Read the model definition and answer for the solid it produces. Units are mm, in the model's axes. Face numbers are marked on the shaded views. A direction names the side the tool comes from. Give positions to 0.01 mm unless a question says otherwise; leave off trailing zeros. Order: outer loops, then holes, each group sorted by start corner. A loop starts at its lowest first (then second) coordinate and runs counter-clockwise, first axis right, second up. Notation, with made-up numbers: (27, -35) - (54, -35) arc R30 cw to (54, -2) - close; hole circle Ø7 at (-7, -33). An arc over 180 degrees is marked (long way). Use a Markdown table: item, result. Add a question column.
1. Consider L1, parallel to X at y = 0, z = 8.3; L2, parallel to Y at x = -41, z = 9 (1 decimal); L3, parallel to X at y = -1.5, z = 1.25. Determine where each line is inside the solid, lowest interval first.
2. Flat-ended cylindrical pins translate along their axes: P1, Ø4.5, axis at x = -16.59, y = 2.11, coming from the +Z side (3 decimals); P2, Ø3.5, axis at x = -41.5, y = -15.5, coming from the -Z side; P3, Ø3, axis at y = 8, z = 12, coming from the -X side. Find the tip coordinate at first contact, or state that the pin passes through.
3. A cutting plane is placed at A-A on z = 9.75. Determine the outline of the cut face in (x, y) (1 decimal).
4. Which of the six approach directions +Z, -Z, +X, -X, +Y, -Y give full straight-line access (tool end or side, diameter ignored) to the marked faces 1, 2, 3 and 4?
5. A cutting plane is placed at B-B on y = 3.5. Determine the outline of the cut face in (x, z) (1 decimal), and give its area (3 significant figures).
6. A cutting plane is placed at C-C on x = -49. Determine the outline of the cut face in (y, z) (1 decimal), and give its area (3 significant figures).
Autodesk Inventor part; units mm, degrees
ref_plane "Work Plane2" through (-20.9694, -2.2685, 9.225) normal (0, 0, -1) x (0.1078, 0.9942, 0)
ref_plane "Work Plane3" through (-49.3551, -24.0887, 15.745) normal (0, 0, -1) x (0, 1, 0)
ref_plane "Work Plane4" through (-51.466, -24.0887, 15.745) normal (0, 0, -1) x (0, 1, 0)
ref_plane "Work Plane5" through (0, 0, 0) normal (0, 0, 1) x (1, 0, 0)
sketch "Sketch1" plane through (0, 0, 0) normal (0, 0, 1) x (1, 0, 0)
  line L0 (-46.1271, -22.5825) -> (-26.1271, -22.5825) construction
  line L1 (-9.7566, 12.6962) -> (-9.7566, -12.6962) construction
  line L2 (-26.1271, 20.28) -> (-46.1271, 20.28) construction
  circle A0 centre (-49.897, 0) radius 1.778
  arc A1 (-26.7903, 1.7468) -> (-25.506, 1.3298) centre (-26.6476, 0) ccw construction
  circle A2 centre (-49.897, 0) radius 1.905
  circle A3 centre (-26.6476, 0) radius 1.905
  line L3 (-52.9366, 6.2882) -> (-52.9366, -15.9368)
  line L4 (-55.4766, 6.2882) -> (-55.4766, -15.9368) construction
  line L5 (-9.7566, -22.5825) -> (-55.4766, -22.5825)
  line L6 (-55.4766, -22.5825) -> (-55.4766, 20.28)
  line L7 (-55.4766, 20.28) -> (-9.7566, 20.28)
  line L8 (-9.7566, 20.28) -> (-9.7566, -22.5825)
  circle A4 centre (-16.5926, 2.1082) radius 2.15 construction
  circle A5 centre (-16.5926, 2.1082) radius 1.9939
  point P0 (0, 0)
  dimension "d0" = 3.81
  dimension "d1" = 3.81
  dimension "d2" = 2.54
  dimension "d3" = 3.9878
ref_plane "Work Plane2" through (-20.9694, -2.2685, 9.225) normal (0, 0, -1) x (0.1078, 0.9942, 0)
extrude "Extrusion1" add sketch "Sketch1" along normal up to surface (9.225 mm away) contours A2 | L5 L6 L7 L8
ref_plane "Work Plane3" through (-49.3551, -24.0887, 15.745) normal (0, 0, -1) x (0, 1, 0)
ref_plane "Work Plane7" through (-55.4766, -22.5825, 9.225) normal (0, 0, 1) x (1, 0, 0)
sketch "Sketch3" plane through (-55.4766, -22.5825, 9.225) normal (0, 0, 1) x (1, 0, 0)
  line L0 (27.2386, 42.8625) -> (7.2386, 42.8625)
  arc A0 (27.2386, 28.0707) -> (27.2386, 14.6543) centre (29.2386, 21.3625) ccw
  line L1 (27.2386, 0) -> (27.2386, 14.6543)
  line L2 (7.2386, 14.6543) -> (7.2386, 0)
  line L3 (7.2386, 0) -> (27.2386, 0)
  arc A1 (7.2386, 14.6543) -> (7.2386, 28.0707) centre (5.2386, 21.3625) ccw
  line L4 (7.2386, 28.0707) -> (7.2386, 42.8625)
  line L5 (0, 42.8625) -> (45.72, 42.8625)
  line L6 (27.2386, 28.0707) -> (27.2386, 42.8625)
  point P0 (55.4766, 22.5825)
ref_plane "Work Plane4" through (-51.466, -24.0887, 15.745) normal (0, 0, -1) x (0, 1, 0)
extrude "Extrusion3" add sketch "Sketch3" along normal up to surface (6.52 mm away)
ref_plane "Work Plane9" through (-55.4766, -22.5825, 9.225) normal (0, 0, 1) x (1, 0, 0)
sketch "Sketch4" plane through (-55.4766, -22.5825, 9.225) normal (0, 0, 1) x (1, 0, 0)
  circle A0 centre (5.5796, 22.5825) radius 1.778
  circle A1 centre (5.5796, 22.5825) radius 1.905
  line L0 (7.2386, 28.0707) -> (7.2386, 42.8625)
  line L1 (7.2386, 42.8625) -> (0, 42.8625)
  line L2 (0, 42.8625) -> (0, 0)
  line L3 (0, 0) -> (7.2386, 0)
  line L4 (7.2386, 0) -> (7.2386, 14.6543)
  arc A2 (7.2386, 14.6543) -> (7.2386, 28.0707) centre (5.2386, 21.3625) ccw
  circle A3 centre (5.5796, 22.5825) radius 1.778
  circle A4 centre (28.829, 22.5825) radius 1.9812
  point P0 (55.4766, 22.5825)
  dimension "d18" = 3.81
hole "Hole1" at (-49.897, 0, 9.225) at (-26.6476, 0, 9.225) direction (0, 0, -1) diameter 3.81 end through all counterbore diameter 10.16 counterbore depth 1.524
ref_plane "Work Plane8" through (-9.7566, -22.5825, 0) normal (1, 0, 0) x (0, 0, -1)
sketch "Sketch6" plane through (-9.7566, -22.5825, 0) normal (1, 0, 0) x (0, 0, -1)
  line L0 (-11.975, 30.2275) -> (-14.475, 30.2275) construction
  line L1 (-11.975, 39.7275) -> (-11.975, 30.2275) construction
  line L2 (31.025, 39.7275) -> (-11.975, 39.7275) construction
  line L3 (31.025, 38.4575) -> (-10.705, 38.4575) construction
  line L4 (-10.705, 32.1075) -> (-10.705, 28.9575) construction
  line L5 (-10.705, 28.9575) -> (-14.475, 28.9575) construction
  line L6 (-10.705, 28.9575) -> (-10.705, 32.1075)
  line L7 (0, 42.8625) -> (0, 0)
  line L8 (0, 32.1075) -> (0, 42.8625)
  line L9 (0, 42.8625) -> (-15.745, 42.8625)
  line L10 (-15.745, 42.8625) -> (-15.745, 28.9575)
  line L11 (-15.745, 28.9575) -> (-10.705, 28.9575)
  line L12 (3.1182, 32.1075) -> (5.3958, 32.1075) construction
  line L13 (-10.705, 32.1075) -> (0, 32.1075)
  point P0 (0, 22.5825)
  point P1 (0, 38.4575)
  dimension "d28" = 1.27
extrude "Extrusion4" cut sketch "Sketch6" against normal through all
sketch "Sketch7" plane through (-48.238, -22.5825, 15.745) normal (0, 0, 1) x (1, 0, 0)
  circle A0 centre (6, 5.3625) radius 2 construction
  circle A1 centre (14, 5.3625) radius 2 construction
  arc A2 (7.4142, 14.7767) -> (4.5858, 11.9483) centre (6, 13.3625) ccw construction
  arc A3 (15.4142, 11.9483) -> (12.5858, 14.7767) centre (14, 13.3625) ccw construction
  point P0 (48.238, 22.5825)
sketch "Sketch9" plane through (0, 0, 0) normal (0, 0, -1) x (-1, 0, 0)
  arc A0 (43.6522, -10.6342) -> (40.8238, -7.8058) centre (42.238, -9.22) ccw construction
  arc A1 (35.6522, -7.8058) -> (32.8238, -10.6342) centre (34.238, -9.22) ccw construction
  circle A2 centre (42.238, -17.22) radius 2 construction
  circle A3 centre (34.238, -17.22) radius 2 construction
  point P0 (0, 0)
hole "Hole2" at (-34.238, -9.22, 0) at (-42.238, -9.22, 0) at (-42.238, -17.22, 0) at (-34.238, -17.22, 0) direction (0, 0, 1) diameter 3.9878 end through all
ref_plane "Work Plane6" through (0, 0, 0) normal (0, 0, -1) x (-1, 0, 0)
sketch "Sketch10" plane through (0, 0, 0) normal (0, 0, -1) x (-1, 0, 0)
  circle A0 centre (34.238, -9.22) radius 1.9939 construction
  circle A1 centre (42.238, -9.22) radius 1.9939 construction
  circle A2 centre (42.238, -17.22) radius 1.9939 construction
  circle A3 centre (34.238, -17.22) radius 1.9939 construction
  circle A4 centre (34.238, -9.22) radius 4.2545 construction
  circle A5 centre (42.238, -9.22) radius 4.2545 construction
  line L0 (34.238, -13.4745) -> (30.5535, -11.3472)
  line L1 (30.5535, -11.3472) -> (30.5535, -7.0927)
  line L2 (30.5535, -7.0927) -> (34.238, -4.9655)
  line L3 (34.238, -4.9655) -> (37.9225, -7.0927)
  line L4 (37.9225, -7.0927) -> (37.9225, -11.3472)
  line L5 (37.9225, -11.3472) -> (34.238, -13.4745)
  circle A6 centre (34.238, -17.22) radius 4.2545 construction
  circle A7 centre (42.238, -17.22) radius 4.2545 construction
  line L6 (38.4925, -17.22) -> (36.3652, -20.9045)
  line L7 (36.3652, -20.9045) -> (32.1107, -20.9045)
  line L8 (32.1107, -20.9045) -> (29.9835, -17.22)
  line L9 (29.9835, -17.22) -> (32.1107, -13.5355)
  line L10 (32.1107, -13.5355) -> (36.3652, -13.5355)
  line L11 (36.3652, -13.5355) -> (38.4925, -17.22)
  line L12 (42.238, -21.4745) -> (38.5535, -19.3472)
  line L13 (38.5535, -19.3472) -> (38.5535, -15.0927)
  line L14 (38.5535, -15.0927) -> (42.238, -12.9655)
  line L15 (42.238, -12.9655) -> (45.9225, -15.0927)
  line L16 (45.9225, -15.0927) -> (45.9225, -19.3472)
  line L17 (45.9225, -19.3472) -> (42.238, -21.4745)
  line L18 (46.4925, -9.22) -> (44.3652, -12.9045)
  line L19 (44.3652, -12.9045) -> (40.1107, -12.9045)
  line L20 (40.1107, -12.9045) -> (37.9835, -9.22)
  line L21 (37.9835, -9.22) -> (40.1107, -5.5355)
  line L22 (40.1107, -5.5355) -> (44.3652, -5.5355)
  line L23 (44.3652, -5.5355) -> (46.4925, -9.22)
  circle A8 centre (16.5926, 2.1082) radius 1.9939 construction
  circle A9 centre (16.5926, 2.1082) radius 4.2545 construction
  line L24 (16.5926, -2.1463) -> (12.9081, -0.019)
  line L25 (12.9081, -0.019) -> (12.9081, 4.2355)
  line L26 (12.9081, 4.2355) -> (16.5926, 6.3627)
  line L27 (16.5926, 6.3627) -> (20.2771, 4.2355)
  line L28 (20.2771, 4.2355) -> (20.2771, -0.019)
  line L29 (20.2771, -0.019) -> (16.5926, -2.1463)
  point P0 (0, 0)
  point P1 (42.238, -13.4745)
  dimension "d38" = 8.509
  dimension "d44" = 8.509
  dimension "d45" = 8.509
  dimension "d48" = 8.509
  dimension "d39" = 8.509
extrude "Extrusion6" cut sketch "Sketch10" against normal blind 5.588 contours L0 L1 L2 L3 L4 L5 | L6 L7 L8 L9 L10 L11 | L12 L13 L14 L15 L16 L17 | L18 L19 L20 L21 L22 L23
extrude "Extrusion7" cut sketch "Sketch10" against normal blind 5.588 contours L24 L25 L26 L27 L28 L29
properties part number "CollectorArmRollerSupportRight"
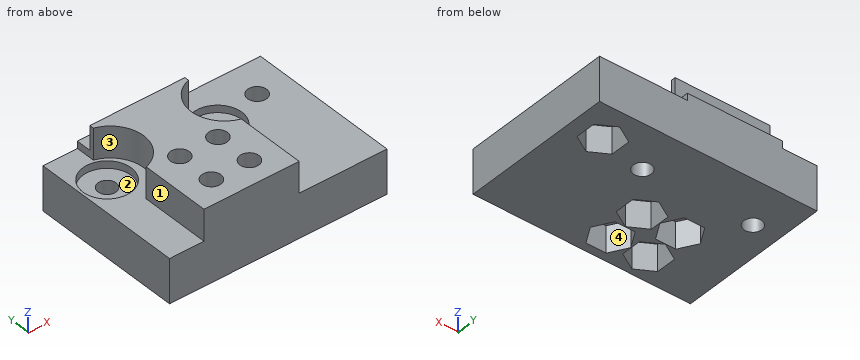
Output values:
| question | item | result |
|---|---|---|
| 1 | L1 | -55.48 to -54.98, -44.82 to -31.73, -21.57 to -9.76 |
| 1 | L2 | -22.6 to -18.8, -15.7 to -10.8, -7.7 to 9.5 |
| 1 | L3 | -55.48 to -51.07, -48.72 to -27.82, -25.47 to -17.71, -15.47 to -9.76 |
| 2 | P1 | z = 9.225 |
| 2 | P2 | z = 5.59 |
| 2 | P3 | x = -48.24 |
| 3 | outline | (-48.2, -22.6) - (-28.2, -22.6) - (-28.2, -7.9) arc R7 cw to (-28.2, 5.5) - (-28.2, 9.5) - (-48.2, 9.5) - (-48.2, 5.5) arc R7 cw to (-48.2, -7.9) - close; hole circle Ø4 at (-42.2, -17.2); hole circle Ø4 at (-42.2, -9.2); hole circle Ø4 at (-34.2, -17.2); hole circle Ø4 at (-34.2, -9.2) |
| 4 | face 1 | +Z, -X, +Y, -Y |
| 4 | face 2 | +Z |
| 4 | face 3 | +Z, -X |
| 4 | face 4 | -Z |
| 5 | outline | (-55.5, 0) - (-20.3, 0) - (-20.3, 5.6) - (-18, 5.6) - (-18, 9.2) - (-23, 9.2) - (-23, 7.7) - (-30.3, 7.7) - (-30.3, 9.2) - (-31.4, 9.2) - (-31.4, 15.7) - (-45.1, 15.7) - (-45.1, 9.2) - (-46.2, 9.2) - (-46.2, 7.7) - (-53.6, 7.7) - (-53.6, 9.2) - (-55.5, 9.2) - close; (-15.2, 5.6) - (-12.9, 5.6) - (-12.9, 0) - (-9.8, 0) - (-9.8, 9.2) - (-15.2, 9.2) - close |
| 5 | area | 437 mm² |
| 6 | outline | (-22.6, 0) - (-1.7, 0) - (-1.7, 7.7) - (-5, 7.7) - (-5, 9.2) - (-22.6, 9.2) - close; (1.7, 0) - (9.5, 0) - (9.5, 9.2) - (5, 9.2) - (5, 7.7) - (1.7, 7.7) - close |
| 6 | area | 255 mm² |
